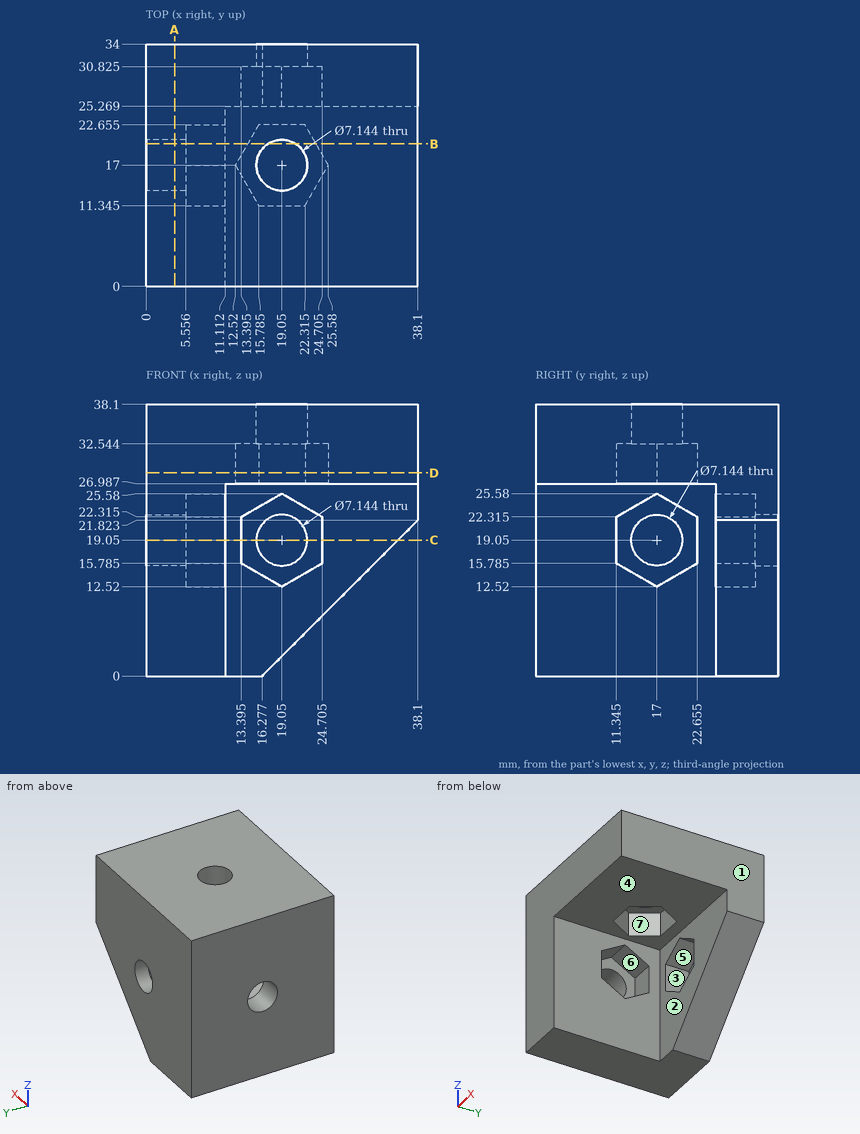
Could you check a few things on this drawing? It's one solid part, dimensions in mm from its lowest x, y, z. A direction names the side the tool comes from. Round coordinates to 2 decimals unless told otherwise and drop trailing zeros. Order: outer loops, then holes, each group sorted by start corner. A loop starts at its lowest first (then second) coordinate and runs counter-clockwise, first axis right, second up. Notation, with made-up numbers: M 53.25,57 L 72.25,57 A12 cw 72.25,73 Z; hole C 72.5,37.5 d6. An arc over 180 degrees is marked long. One line per item, written item: value.
(1) Imagine slicing it at B-B (y = 20). Write out the boundary of the cut face in (x, z).
Ans:
outline: M 0,0 L 11.11,0 L 11.11,14.25 L 5.56,14.25 L 5.56,17.11 L 0,17.11 Z; M 0,20.99 L 5.56,20.99 L 5.56,23.85 L 11.11,23.85 L 11.11,26.99 L 14.25,26.99 L 14.25,32.54 L 17.11,32.54 L 17.11,38.1 L 0,38.1 Z; M 20.99,32.54 L 23.85,32.54 L 23.85,26.99 L 38.1,26.99 L 38.1,38.1 L 20.99,38.1 Z
(2) Imagine slicing it at C-C (z = 19.05). Write out the boundary of the cut face in (x, y) (1 decimal), and give its area (3 significant figures).
Ans:
outline: M 0,0 L 11.1,0 L 11.1,11.3 L 5.6,11.3 L 5.6,13.4 L 0,13.4 Z; M 0,20.6 L 5.6,20.6 L 5.6,22.7 L 11.1,22.7 L 11.1,25.3 L 13.4,25.3 L 13.4,30.8 L 15.5,30.8 L 15.5,34 L 0,34 Z; M 22.6,30.8 L 24.7,30.8 L 24.7,25.3 L 35.3,25.3 L 35.3,34 L 22.6,34 Z
area: 401 mm^2
(3) Imagine slicing it at A-A (x = 4). Write out the boundary of the cut face in (y, z), and give its area (3 significant figures).
Ans:
outline: M 0,0 L 34,0 L 34,38.1 L 0,38.1 Z; hole C 17,19.05 d7.14
area: 1,260 mm^2
(4) If we mould it in two halves opening along X, with no side actions, what happens to the marked faces 1, 2 and 3? For each: released by +X, released by -X, zero draft, split by the parting line, or undercut.
Ans:
face 1: released by +X
face 2: zero draft
face 3: undercut
(5) Which directions (+Z, -Z, +X, -X, +Y, -Y) give clear straight access to the entire face, cutting with the end or side of a thin tool? Please do the marked faces 4, 5, 6 and 7.
Ans:
face 4: -Z, +X, -Y
face 5: -Y
face 6: +X
face 7: -Z
(6) I'm going to push flat-ended pins straight in: P1, Ø3.5, axis at y = 14.5, z = 17, coming from the +X side; P2, Ø12.5, axis at y = 7.5, z = 17, coming from the +X side; P3, Ø20, axis at x = 28.5, y = 6.5, coming from the -Z side. Where does each tip first touch, or does it pass through?
Ans:
P1: stops at x = 5.56
P2: stops at x = 11.11
P3: stops at z = 26.99
(7) I need wall thicknesses on line 1 along Y through (x, z) = (1.4, 19.05); line 2 along Z through (x, y) = (19.5, 8); line 3 along Y through (x, z) = (32.5, 19). Which ranges of each line are inside material? Lowest first, please. Write a range as from..to.
Ans:
line 1: y = 0..13.43, 20.57..34
line 2: z = 26.99..38.1
line 3: y = 25.27..34
(8) Imagine slicing it at D-D (z = 28.5). Write out the boundary of the cut face in (x, y) (1 decimal).
Ans:
outline: M 0,0 L 38.1,0 L 38.1,34 L 0,34 Z; hole M 12.5,17 L 15.8,11.3 L 22.3,11.3 L 25.6,17 L 22.3,22.7 L 15.8,22.7 Z
